Work out the finished part from the listing and answer in its coordinate system (mm). A direction names the side the tool comes from. Round coordinates to 2 decimals unless told otherwise and drop trailing zeros. Write each loop counter-clockwise with the first axis right and the second up, starting at its lowest first coordinate (ties: lowest second). Pieces come first, ordered by that corner, then holes. Notation, with made-up numbers: (83.5, -30) - (118.5, -30) arc R14 ccw to (118.5, -9) - close; hole circle Ø4 at (50, 64). An arc over 180 degrees is marked (long way). Answer as a JSON object with one key per item and string values.
```python
from build123d import *

# Parameters (mm, degrees)
CROQUIS1_W              = 42
CROQUIS1_H              = 42
SALIENTE_EXTRUIR1_DEPTH = 22
CROQUIS2_W              = 25
CROQUIS2_H              = 25
CROQUIS2_W_2            = 22.6
CROQUIS2_H_2            = 22.6
CORTAR_EXTRUIR1_DEPTH   = 15
CROQUIS3_R              = 5
CORTAR_EXTRUIR2_DEPTH   = 37.959437225
CROQUIS4_R              = 11
CORTAR_EXTRUIR3_DEPTH   = 3.5
CROQUIS5_R              = 10
CORTAR_EXTRUIR4_DEPTH   = 9
CROQUIS6_R              = 2
CORTAR_EXTRUIR5_DEPTH   = 37.959437225
REDONDEO1_R             = 4
CROQUIS7_R              = 2.5
CORTAR_EXTRUIR7_DEPTH   = 52.85556865
CHAFL_N1_SIZE           = 2


with BuildPart() as part:
    # Croquis1 → Saliente-Extruir1 (new body)
    with BuildSketch(Plane.XY):
        Rectangle(CROQUIS1_W, CROQUIS1_H)
    extrude(amount=SALIENTE_EXTRUIR1_DEPTH)

    # Croquis2 → Cortar-Extruir1 (cut)
    with BuildSketch(Plane(origin=(0, 0, 0), x_dir=(-1, 0, 0), z_dir=(0, 0, -1))):
        Rectangle(CROQUIS2_W, CROQUIS2_H)
        Rectangle(CROQUIS2_W_2, CROQUIS2_H_2, mode=Mode.SUBTRACT)
    extrude(amount=-CORTAR_EXTRUIR1_DEPTH, mode=Mode.SUBTRACT)

    # Croquis3 → Cortar-Extruir2 (cut, through all)
    with BuildSketch(Plane.XY.offset(22)):
        Circle(CROQUIS3_R)
    extrude(amount=-CORTAR_EXTRUIR2_DEPTH, mode=Mode.SUBTRACT)

    # Croquis4 → Cortar-Extruir3 (cut)
    with BuildSketch(Plane.XY.offset(22)):
        Circle(CROQUIS4_R)
    extrude(amount=-CORTAR_EXTRUIR3_DEPTH, mode=Mode.SUBTRACT)

    # Croquis5 → Cortar-Extruir4 (cut)
    with BuildSketch(Plane.XY.offset(18.5)):
        Circle(CROQUIS5_R)
    extrude(amount=-CORTAR_EXTRUIR4_DEPTH, mode=Mode.SUBTRACT)

    # Croquis6 → Cortar-Extruir5 (cut, through all)
    with BuildSketch(Plane(origin=(0, 0, 0), x_dir=(-1, 0, 0), z_dir=(0, 0, -1))):
        with Locations((17, 17)):
            Circle(CROQUIS6_R)
        with Locations((-17, 17)):
            Circle(CROQUIS6_R)
        with Locations((-17, -17)):
            Circle(CROQUIS6_R)
        with Locations((17, -17)):
            Circle(CROQUIS6_R)
    extrude(amount=-CORTAR_EXTRUIR5_DEPTH, mode=Mode.SUBTRACT)

    # Redondeo1
    redondeo1_edges = [part.edges().sort_by_distance(p)[0] for p in [
        (21, -21, 11),
        (-21, -21, 11),
        (-21, 21, 11),
        (21, 21, 11),
    ]]
    fillet(redondeo1_edges, radius=REDONDEO1_R)

    # Croquis7 → Cortar-Extruir7 (cut, through all)
    with BuildSketch(Plane(origin=(21, 0, 0), x_dir=(0, 0, -1), z_dir=(1, 0, 0))):
        with Locations(Location((-8, 0, 0), (0, 0, 126.869897646))):
            Circle(CROQUIS7_R)
    extrude(amount=-CORTAR_EXTRUIR7_DEPTH, mode=Mode.SUBTRACT)

    # Chaflán1
    chafl_n1_edges = [part.edges().sort_by_distance(p)[0] for p in [
        (-21, -2, 6.5),
        (21, -2, 6.5),
    ]]
    chamfer(chafl_n1_edges, length=CHAFL_N1_SIZE)


solid = part.part
```
Item 1: A cutting plane is placed at D-D (y = 8). Write down the section's boundary in (x, z), and give its area (3 significant figures).
Results found:
{"outline": "(-21, 0) - (-12.5, 0) - (-12.5, 15) - (-11.3, 15) - (-11.3, 0) - (11.3, 0) - (11.3, 15) - (12.5, 15) - (12.5, 0) - (21, 0) - (21, 22) - (7.55, 22) - (7.55, 18.5) - (6, 18.5) - (6, 9.5) - (-6, 9.5) - (-6, 18.5) - (-7.55, 18.5) - (-7.55, 22) - (-21, 22) - close", "area": "727 mm²"}
Item 2: A cutting plane is placed at B-B (z = 8). Give the number of separate pieces and of enclosed holes in the cut face, and give its area (3 significant figures).
Results found:
{"separate pieces": "4", "enclosed holes": "4", "area": "1,350 mm²"}
Item 3: For faces 5 (the cylindrical face through (8.64, 1.03, 5.72)), 6 (the cylindrical face through (9.54, 3, 14.06)), 7 (the flat face through (0, 11.3, 7)), determine the directions among +Z, -Z, +X, -X, +Y, -Y from which every point of the face is accessible in a straight line to the end or side of a thin tool.
Results found:
{"face 5": "+X, -X", "face 6": "+Z", "face 7": "-Z"}
Item 4: Consider line 1 along Y through (x, z) = (17, 15.25); line 2 along Y through (x, z) = (-17, 7.75); line 3 along Y through (x, z) = (0, 7). Determine where each line is inside the solid, lowest interval first.
Results found:
{"line 1": "-21 to -19, -15 to 15, 19 to 21", "line 2": "-21 to -19, -15 to -2.49, 2.49 to 15, 19 to 21", "line 3": "-21 to -12.5, -11.3 to -5, 5 to 11.3, 12.5 to 21"}
Item 5: Determine the mould class of faces 1 (the flat face through (12.5, -3, 7)), 2 (the flat face through (21, 0, 13)), 3 (the flat face through (0, 21, 11)), 4 (the cylindrical face through (-17, 19, 11)) for opening direction X: pulls with the +X half, pulls with the -X half, needs draft (parallel to the pull), parting line crosses it, or undercut.
Results found:
{"face 1": "undercut", "face 2": "pulls with the +X half", "face 3": "needs draft", "face 4": "undercut"}
Item 6: Each of these flat-tipped pins is pushed along its axis until it touches: P1, Ø4.5, axis at y = -2, z = 8, coming from the -X side; P2, Ø4, axis at x = 4, y = 4.5, coming from the +Z side. Where does it stop, or does it pass through?
Results found:
{"P1": "x = -20.75", "P2": "z = 9.5"}
Item 7: A cutting plane is placed at A-A (z = 14.25). Write down the section's boundary in (x, y), and give its area (3 significant figures).
Results found:
{"outline": "(-21, -17) arc R4 ccw to (-17, -21) - (17, -21) arc R4 ccw to (21, -17) - (21, 17) arc R4 ccw to (17, 21) - (-17, 21) arc R4 ccw to (-21, 17) - close; (-11.3, -11.3) - (11.3, -11.3) - (11.3, 11.3) - (-11.3, 11.3) - close; hole circle Ø4 at (-17, -17); hole circle Ø4 at (-17, 17); hole (-12.5, -12.5) - (12.5, -12.5) - (12.5, 12.5) - (-12.5, 12.5) - close; hole circle Ø20 at (0, 0); hole circle Ø4 at (17, -17); hole circle Ø4 at (17, 17)", "area": "1,270 mm²"}
